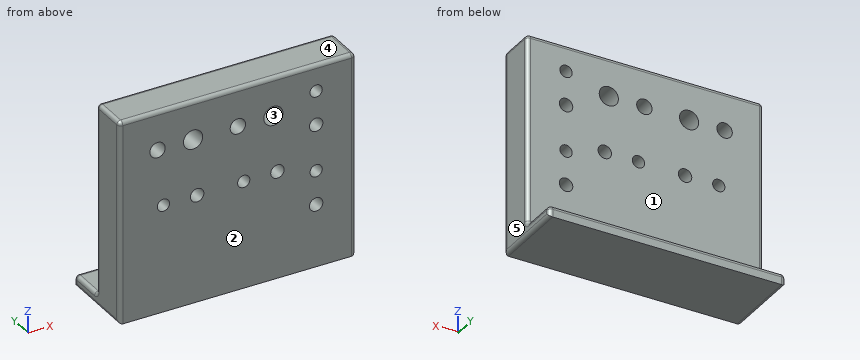
from build123d import *

# Parameters (mm, degrees)
F0_W          = 100
F0_H          = 5
F1_DEPTH      = 3
F2_W          = 100
F2_H          = 10
F3_DEPTH      = 50
F4_R          = 1.6
F4_R_2        = 1.75
F4_R_3        = 2.5
F4_R_4        = 2
F5_DEPTH      = 50
F7_DEPTH      = 50
F7_DEPTH_BACK = 25
F8_R          = 1


with BuildPart() as f1:
    # F0 (on Top) → F1 (new body)
    with BuildSketch(Plane.XY):
        with Locations((0, 12.6435890049)):
            Rectangle(F0_W, F0_H)
        with Locations((0, 7.6435890049)):
            Rectangle(F0_W, F0_H)
        with Locations((0, 2.6435890049)):
            Rectangle(F0_W, F0_H)
        with Locations((0, -2.3564109951)):
            Rectangle(F0_W, F0_H)
    extrude(amount=F1_DEPTH)

    # F2 (on face) → F3 (join)
    with BuildSketch(Plane.XY.offset(3)):
        with Locations((0, 0.1435890049)):
            Rectangle(F2_W, F2_H)
    extrude(amount=F3_DEPTH)

    # F4 (on face) → F5 (cut)
    with BuildSketch(Plane.XZ.offset(4.8564109951)):
        with Locations((0, 28)):
            Circle(F4_R)
        with Locations((39.7706801567, 25.1996132218)):
            Circle(F4_R)
        with Locations((8.7829349406, 28)):
            Circle(F4_R_2)
        with Locations((39.7706801567, 37.2641024557)):
            Circle(F4_R_2)
        with Locations((20.9091, 28)):
            Circle(F4_R)
        with Locations((29.6920349406, 28)):
            Circle(F4_R_2)
        with Locations((39.7706801567, 46.1087132218)):
            Circle(F4_R)
        with Locations((39.7706801567, 16.3550024557)):
            Circle(F4_R_2)
        with Locations((7.7257619488, 42.9009612363)):
            Circle(F4_R_3)
        with Locations((28.6348619488, 42.9009612363)):
            Circle(F4_R_3)
        with Locations((-1.5212555765, 42.9009612363)):
            Circle(F4_R_4)
        with Locations((19.3878444235, 42.9009612363)):
            Circle(F4_R_4)
    extrude(amount=-F5_DEPTH, mode=Mode.SUBTRACT)

    # F6 (on face) → F7 (cut, two sides)
    with BuildSketch(Plane.XZ.offset(4.8564109951)) as f7_sk:
        Polygon((-50, 53), (-11.575919576, 53), (-11.575919576, 62.5623986125), (-61.6087988019, 62.5623986125), (-61.6087988019, -15.408792533), (-11.575919576, -17.8658775985), (-11.575919576, 0), (-50, 0), align=None)
        Polygon((-11.575919576, 0), (-11.575919576, 49.896787852), (-11.575919576, 53), (-50, 53), (-50, 0), align=None)
    extrude(amount=-F7_DEPTH, mode=Mode.SUBTRACT)
    extrude(f7_sk.sketch, amount=F7_DEPTH_BACK, mode=Mode.SUBTRACT)

    # F8
    f8_edges = [f1.edges().sort_by_distance(p)[0] for p in [
        (50, -4.856411, 26.5),
        (50, 0.143589, 53),
        (50, 5.143589, 28),
        (50, 10.143589, 3),
        (50, 15.143589, 1.5),
        (50, 5.143589, 0),
        (-11.57592, 0.143589, 53),
        (19.21204, 5.143589, 53),
        (19.21204, -4.856411, 53),
        (-11.57592, 5.143589, 0),
        (-11.57592, -4.856411, 26.5),
        (-11.57592, 5.143589, 28),
        (-11.57592, 10.143589, 3),
        (-11.57592, 15.143589, 1.5),
        (19.21204, 5.143589, 3),
        (19.21204, 15.143589, 3),
    ]]
    fillet(f8_edges, radius=F8_R)


solid = f1.part
Check sheet for the modelled part. Datum: model origin and axes. Units: mm. Face numbers are marked on the shaded views. A direction names the side the tool comes from. Give positions to 0.01 mm unless a question says otherwise; leave off trailing zeros. Order: outer loops, then holes, each group sorted by start corner. A loop starts at its lowest first (then second) coordinate and runs counter-clockwise, first axis right, second up. Notation, with made-up numbers: M -22,-33.75 L -11,-33.75 A14 cw -11,-20.75 Z; hole C -17.75,4 d11. An arc over 180 degrees is marked long. Answer as CSV lines item,"result". Start each with the question number.
Item 1: Tool access check on the marked faces 1 and 2. Record the directions out of +Z, -Z, +X, -X, +Y, -Y that give a thin tool (end or side, any length) a straight path to the whole face; none if there is none.
Item 2: Mould release check, pull along Z, two halves, no side actions. Record for the marked faces 3, 4 and 5: +Z half, -Z half, draft (parallel to the pull), parting line (faces both ways), or undercut.
Item 3: Cross-section at C-C on y = 3. State how many separate pieces and enclosed holes the cut face has, plus the area to 3 significant figures.
Item 4: Cross-section at A-A on z = 28. Enter the section's corners in (x, y).
Item 5: Cross-section at D-D on x = -2.5. Enter the section's corners in (y, z).
Item 6: Thickness scan on line 1 (Z direction, x = 29, y = -0.5); line 2 (Y direction, x = 46.5, z = 18); line 3 (Z direction, x = 44, y = 9.5). Record the ranges inside material, lowest first. Write a range as [from, to].
Item 7: Cross-section at B-B on x = 16. Enter the section's corners in (y, z), plus the area to 3 significant figures.
Item 8: Gauge pin test, flat ends, axial feed: P1, Ø8, axis at x = 7.73, z = 42.9, coming from the +Y side; P2, Ø4, axis at x = 19, y = 10, coming from the +Z side. Record the tip position at first contact, or that the pin passes through.
Established:
1,face 1,"+Z, +X, -X, +Y"
1,face 2,"+Z, -Z, +X, -X, -Y"
2,face 3,"undercut"
2,face 4,"+Z half"
2,face 5,"draft"
3,separate pieces,"1"
3,enclosed holes,"12"
3,area,"3,130 mm^2"
4,outline,"M -11.58,-3.86 A1 ccw -10.58,-4.86 L -1.6,-4.86 L -1.6,5.14 L -10.58,5.14 A1 ccw -11.58,4.14 Z; M 1.6,-4.86 L 7.03,-4.86 L 7.03,5.14 L 1.6,5.14 Z; M 10.53,-4.86 L 19.31,-4.86 L 19.31,5.14 L 10.53,5.14 Z; M 22.51,-4.86 L 27.94,-4.86 L 27.94,5.14 L 22.51,5.14 Z; M 31.44,-4.86 L 49,-4.86 A1 ccw 50,-3.86 L 50,4.14 A1 ccw 49,5.14 L 31.44,5.14 Z"
5,outline,"M -4.86,0 L 15.14,0 L 15.14,2 A1 ccw 14.14,3 L 6.14,3 A1 cw 5.14,4 L 5.14,41.16 L -4.86,41.16 Z; M -4.86,44.65 L 5.14,44.65 L 5.14,52 A1 ccw 4.14,53 L -3.86,53 A1 ccw -4.86,52 Z"
6,line 1,"z = [0, 26.39], [29.61, 40.43], [45.37, 53]"
6,line 2,"y = [-4.86, 5.14]"
6,line 3,"z = [0, 3]"
7,outline,"M -4.86,0 L 15.14,0 L 15.14,2 A1 ccw 14.14,3 L 6.14,3 A1 cw 5.14,4 L 5.14,52 A1 ccw 4.14,53 L -3.86,53 A1 ccw -4.86,52 Z"
7,area,"560 mm^2"
8,P1,"stops at y = 5.14"
8,P2,"stops at z = 3"
